CAD build for the part. Positions are in the model's coordinates, mm. A direction names the side the tool comes from. Give positions to 0.01 mm unless a question says otherwise; leave off trailing zeros. Write each loop counter-clockwise with the first axis right and the second up, starting at its lowest first coordinate (ties: lowest second). Pieces come first, ordered by that corner, then holes. Notation, with made-up numbers: (-22.5, 70.5) - (-15.5, 70.5) arc R34 ccw to (-15.5, 103.5) - close; hole circle Ø10 at (36.25, 35). An arc over 180 degrees is marked (long way). Put each result on its own line as item: value. Start each with the question number.
1. Cut at C-C on y = -21. List the corners of the cut face in (x, z), and give its area (3 significant figures).
2. Cut at B-B on x = 60.75. List the corners of the cut face in (y, z), and give its area (3 significant figures).
3. Wall check: line 1 (Y direction, x = 37, z = 29.3); line 2 (X direction, y = -52, z = 6); line 3 (Z direction, x = 67.5, y = -45.5). Give the ranges that are in metal, low to high.
4. Tool access for faces 4 (the cylindrical face through (35.959, -37.068, 28.521)), 5 (the cylindrical face through (20.27, -24.15, 47.63)), 6 (the flat face through (37, -13, 40)): list every direction of +Z, -Z, +X, -X, +Y, -Y with a clear straight run to the whole face (end or side of a thin tool).
5. Mould opens along X. For faces 1 (the cylindrical face through (63.06, -8.21, 28.52)), 2 (the flat face through (37, -23, 50)), 3 (the flat face through (7, -28, 44)) say: +X half, -X half, draft (parallel to the pull), parting line (faces both ways), or undercut.
6. Cut at A-A on z = 40. List the corners of the cut face in (x, y), and give its area (3 significant figures).
7. Cut at D-D on x = 32.5. List the corners of the cut face in (y, z).
8. Drop flat-ended pins along their axis: pin 1 (1 mm diameter, centred on x = 46, z = 39.5, fed in from -Y); pin 2 (5.5 mm diameter, centred on x = 56.5, y = -23, fed in from +Z); pin 3 (10 mm diameter, centred on x = 35, y = -50.5, fed in from +Z). Give the stop position or say it passes through.
from build123d import *

# Parameters (mm, degrees)
F1_DEPTH  = 83
F2_R      = 2.5
F3_DEPTH  = 30.001
F4_R      = 8
F4_R_2    = 6
F5_DEPTH  = 30.001
F6_R      = 3
F7_DEPTH  = 74.001
F8_W      = 60
F8_H      = 20
F9_DEPTH  = 20
F10_R     = 6
F11_DEPTH = 67.001
F12_R     = 3
F13_DEPTH = 4.8048476773


with BuildPart() as f1:
    # F0 (on Front) → F1 (new body)
    with BuildSketch(Plane.XZ):
        with BuildLine():
            Line((0, 27), (0, 0))
            Line((0, 0), (3, 0))
            Line((3, 0), (3, 25.5))
            ThreePointArc((3, 25.5), (3.4393398282, 26.5606601718), (4.5, 27))
            Line((4.5, 27), (69.5, 27))
            ThreePointArc((69.5, 27), (70.5606601718, 26.5606601718), (71, 25.5))
            Line((71, 25.5), (71, 0))
            Line((71, 0), (74, 0))
            Line((74, 0), (74, 27))
            ThreePointArc((74, 27), (73.1213203436, 29.1213203436), (71, 30))
            Line((71, 30), (3, 30))
            ThreePointArc((3, 30), (0.8786796564, 29.1213203436), (0, 27))
        make_face()
    extrude(amount=F1_DEPTH)

    # F2 (on face) → F3 (cut, through all)
    with BuildSketch(Plane.XY.offset(30)):
        with Locations((13.25, -7.25)):
            Circle(F2_R)
        with Locations((60.75, -7.25)):
            Circle(F2_R)
        with Locations((60.75, -75.75)):
            Circle(F2_R)
        with Locations((13.25, -75.75)):
            Circle(F2_R)
    extrude(amount=-F3_DEPTH, mode=Mode.SUBTRACT)

    # F4 (on face) → F5 (cut, through all)
    with BuildSketch(Plane.XY.offset(30)):
        with Locations((37, -45)):
            Circle(F4_R)
        with Locations((56, -48)):
            Circle(F4_R_2)
        with Locations((53, -64)):
            Circle(F4_R_2)
        with Locations((37, -63.5)):
            Circle(F4_R_2)
        with Locations((18, -48)):
            Circle(F4_R_2)
    extrude(amount=-F5_DEPTH, mode=Mode.SUBTRACT)

    # F6 (on face) → F7 (cut, through all)
    with BuildSketch(Plane(origin=(0, 0, 0), x_dir=(0, -1, 0), z_dir=(-1, 0, 0))):
        with Locations((7, 7)):
            Circle(F6_R)
        with Locations((76, 7)):
            Circle(F6_R)
    extrude(amount=-F7_DEPTH, mode=Mode.SUBTRACT)

    # F8 (on face) → F9 (join)
    with BuildSketch(Plane.XY.offset(30)):
        with Locations((37, -23)):
            Rectangle(F8_W, F8_H)
    extrude(amount=F9_DEPTH)

    # F10 (on face) → F11 (cut, through all)
    with BuildSketch(Plane(origin=(7, 0, 0), x_dir=(0, -1, 0), z_dir=(-1, 0, 0))):
        with Locations((23, 40)):
            Circle(F10_R)
    extrude(amount=-F11_DEPTH, mode=Mode.SUBTRACT)

    # F12 (on face) → F13 (cut, through all)
    with BuildSketch(Plane.XY.offset(50)):
        with Locations((17.5, -23)):
            Circle(F12_R)
        with Locations((56.5, -23)):
            Circle(F12_R)
    extrude(amount=-F13_DEPTH, mode=Mode.SUBTRACT)


solid = f1.part
Report:
1. outline: (0, 0) - (3, 0) - (3, 25.5) arc R1.5 cw to (4.5, 27) - (69.5, 27) arc R1.5 cw to (71, 25.5) - (71, 0) - (74, 0) - (74, 27) arc R3 ccw to (71, 30) - (67, 30) - (67, 34.34) - (7, 34.34) - (7, 30) - (3, 30) arc R3 ccw to (0, 27) - close; (7, 45.66) - (15.26, 45.66) - (15.26, 50) - (7, 50) - close; (19.74, 45.66) - (54.26, 45.66) - (54.26, 50) - (19.74, 50) - close; (58.74, 45.66) - (67, 45.66) - (67, 50) - (58.74, 50) - close
1. area: 863 mm²
2. outline: (-83, 27) - (-78.25, 27) - (-78.25, 30) - (-83, 30) - close; (-73.25, 27) - (-51.67, 27) - (-51.67, 30) - (-73.25, 30) - close; (-44.33, 27) - (-9.75, 27) - (-9.75, 30) - (-13, 30) - (-13, 50) - (-33, 50) - (-33, 30) - (-44.33, 30) - close; (-4.75, 27) - (0, 27) - (0, 30) - (-4.75, 30) - close; hole circle Ø12 at (-23, 40)
2. area: 484 mm²
3. line 1: y = -83 to -69.5, -57.5 to -53, -37 to 0
3. line 2: x = 0 to 3, 71 to 74
3. line 3: z = 27 to 30
4. face 4: +Z, -Z
4. face 5: +Z
4. face 6: +Z, +X, -X, +Y
5. face 1: undercut
5. face 2: draft
5. face 3: -X half
6. outline: (7, -33) - (67, -33) - (67, -29) - (7, -29) - close; (7, -17) - (67, -17) - (67, -13) - (7, -13) - close
6. area: 480 mm²
7. outline: (-83, 27) - (-67.47, 27) - (-67.47, 30) - (-83, 30) - close; (-59.53, 27) - (-51.61, 27) - (-51.61, 30) - (-59.53, 30) - close; (-38.39, 27) - (0, 27) - (0, 30) - (-13, 30) - (-13, 50) - (-33, 50) - (-33, 30) - (-38.39, 30) - close; hole circle Ø12 at (-23, 40)
8. pin 1: stops at y = -33
8. pin 2: stops at z = 34.67
8. pin 3: stops at z = 30
